Geometry: final body of the model. Coordinates: model frame, mm. A direction names the side the tool comes from. Give positions to 0.01 mm unless a question says otherwise; leave off trailing zeros. Loops run counter-clockwise (first coordinate to the right, second up) from the corner with the lowest first, then second, coordinate; pieces in that order, holes last. Notation, with made-up numbers: M 46,12 L 56,12 A25 cw 56,24 Z; hole C 15.5,39 d10. An arc over 180 degrees is marked long. Put each result on its own line as item: value.
Autodesk Inventor part; units mm, degrees
ref_plane "YZ Plane" through (0, 0, 0) normal (1, 0, 0) x (0, 1, 0)
ref_plane "XZ Plane" through (0, 0, 0) normal (0, 1, 0) x (-1, 0, 0)
ref_plane "XY Plane" through (0, 0, 0) normal (0, 0, 1) x (1, 0, 0)
sketch "Szkic1" plane through (0, 0, 0) normal (0, 0, 1) x (1, 0, 0)
  line L0 (-17.1731, 6.2025) -> (7.8269, 6.2025)
  line L1 (7.8269, 6.2025) -> (7.8269, -4.7975)
  line L2 (7.8269, -4.7975) -> (-17.1731, -4.7975)
  line L3 (-17.1731, -4.7975) -> (-17.1731, 6.2025)
  point P0 (0, 0)
  point P1 (-13.6731, 0.7025)
  point P2 (4.3269, 0.7025)
  dimension "d0" = 25
  dimension "d1" = 11
  dimension "d2" = 5.5
  dimension "d3" = 5.5
  dimension "d4" = 3.5
  dimension "d5" = 3.5
extrude "Wyciągnięcie proste1" add sketch "Szkic1" along normal blind 2
hole "Otwór1" at (-13.6731, 0.7025, 0) at (4.3269, 0.7025, 0) direction (0, 0, 1) diameter 3 end through all
fillet "Zaokrąglenie1" radius 3 4 edges at (-17.1731, 6.2025, 1) (-17.1731, -4.7975, 1) (7.8269, 6.2025, 1) (7.8269, -4.7975, 1)
sketch "Szkic3" plane through (0, 0, 2) normal (0, 0, 1) x (1, 0, 0)
  arc A0 (4.8269, -4.7975) -> (7.8269, -1.7975) centre (4.8269, -1.7975) ccw
  line L0 (7.8269, -1.7975) -> (7.8269, 3.2025)
  arc A1 (7.8269, 3.2025) -> (4.8269, 6.2025) centre (4.8269, 3.2025) ccw
  line L1 (4.8269, 6.2025) -> (-14.1731, 6.2025)
  arc A2 (-14.1731, 6.2025) -> (-17.1731, 3.2025) centre (-14.1731, 3.2025) ccw
  line L2 (-17.1731, 3.2025) -> (-17.1731, -1.7975)
  arc A3 (-17.1731, -1.7975) -> (-14.1731, -4.7975) centre (-14.1731, -1.7975) ccw
  line L3 (-14.1731, -4.7975) -> (4.8269, -4.7975)
  circle A4 centre (-13.6731, 0.7025) radius 1.5
  circle A5 centre (4.3269, 0.7025) radius 1.5
  line L4 (-14.1731, 8.2025) -> (4.8269, 8.2025)
  arc A6 (9.8269, 3.2025) -> (4.8269, 8.2025) centre (4.8269, 3.2025) ccw
  line L5 (9.8269, 3.2025) -> (9.8269, -1.7975)
  arc A7 (4.8269, -6.7975) -> (9.8269, -1.7975) centre (4.8269, -1.7975) ccw
  line L6 (4.8269, -6.7975) -> (-14.1731, -6.7975)
  arc A8 (-19.1731, -1.7975) -> (-14.1731, -6.7975) centre (-14.1731, -1.7975) ccw
  line L7 (-19.1731, -1.7975) -> (-19.1731, 3.2025)
  arc A9 (-14.1731, 8.2025) -> (-19.1731, 3.2025) centre (-14.1731, 3.2025) ccw
  point P0 (0, 0)
  dimension "d16" = 2
extrude "Wyciągnięcie proste2" add sketch "Szkic3" along normal blind 2 contours L3 A3 L2 A2 L1 A1 L0 A0 | L4 A6 L5 A7 L6 A8 L7 A9
fillet "Zaokrąglenie2" radius 1.7 16 edges at (8.3624, -5.333, 2) (-4.6731, -6.7975, 2) (-17.7087, -5.333, 2) (-19.1731, 0.7025, 2) (-17.7087, 6.7381, 2) (-4.6731, 8.2025, 2) (8.3624, 6.7381, 2) (9.8269, 0.7025, 2) (6.9482, 5.3238, 2) (-4.6731, 6.2025, 2) (-16.2944, 5.3238, 2) (-17.1731, 0.7025, 2) (-16.2944, -3.9188, 2) (-4.6731, -4.7975, 2) (6.9482, -3.9188, 2) (7.8269, 0.7025, 2)
properties part number "3DP_ABS_Y_Axis_Belt_Mount_Spacer"
Item 1: Pin query (flat end, axial travel): pin 1 Ø0.7 at (y, z) = (0.5, 0.5) entering from +X; pin 2 Ø0.7 at (y, z) = (-0.5, 0) entering from -X. Return the tip coordinate at first contact, or that it passes through.
Output values:
pin 1: x = 7.85
pin 2: x = -17.17
Item 2: Section B-B on y = 1.25. Count the separate pieces of the cut face and the enclosed holes in it, then the cut area to 3 significant figures.
Output values:
separate pieces: 3
enclosed holes: 0
area: 85.1 mm²
Item 3: Set-up query: faces 1 (the cylindrical face through (6.97, 5.3, 0.31)), 2 (the cylindrical face through (6.925, -3.942, 0.305)), 3 (the cylindrical face through (-16.318, -3.895, 0.305)), 4 (the cylindrical face through (-18.91, 0.67, 2.79)), 5 (the cylindrical face through (-16.27, 5.35, 0.31)). Return all of +Z, -Z, +X, -X, +Y, -Y with unobstructed straight access to the full face (end or side cutting, diameter ignored); none if empty.
Output values:
face 1: -Z, +X, +Y
face 2: -Z, +X, -Y
face 3: -Z, -X, -Y
face 4: -Z, -X, +Y, -Y
face 5: -Z, -X, +Y
Item 4: Line query: probe 1 along X at (y, z) = (1, 2.9); probe 2 along Y at (x, z) = (-12.75, 3.05); probe 3 along Y at (x, z) = (5, 3.2). Output: solid intervals per line, ascending. Write a range as [from, to].
Output values:
probe 1: [-18.97, -15.14], [-12.2, 2.86], [5.8, 9.63]
probe 2: [-6.67, -0.48], [1.88, 8.07]
probe 3: [-6.72, -0.64], [2.04, 8.12]
Item 5: Section A-A on z = 2.9. Output: boundary loops of the cut face in (x, y), then the cut area to 3 significant figures.
Output values:
outline: M -18.97,-1.8 A4.8 ccw -14.17,-6.6 L 4.83,-6.6 A4.8 ccw 9.63,-1.8 L 9.63,3.2 A4.8 ccw 4.83,8 L -14.17,8 A4.8 ccw -18.97,3.2 Z; hole C -13.67,0.7 d3; hole C 4.33,0.7 d3
area: 384 mm²
